Check sheet for the modelled part. Datum: model origin and axes. Units: mm. Coordinates: 2 decimals unless noted, no trailing zeros. Order: outer loops, then holes, each group sorted by start corner. A loop starts at its lowest first (then second) coordinate and runs counter-clockwise, first axis right, second up. Notation, with made-up numbers: (16.25, -34.5) -> (43.25, -34.5) arc R15 ccw to (43.25, -23.5) -> close; hole circle Ø1 at (26, 54.25). An arc over 180 degrees is marked (long way). Put each result on its own line as item: value. Start each with the question number.
Autodesk Inventor part; units mm, degrees
ref_plane "YZ Plane" through (0, 0, 0) normal (1, 0, 0) x (0, 1, 0)
ref_plane "XZ Plane" through (0, 0, 0) normal (0, 1, 0) x (-1, 0, 0)
ref_plane "XY Plane" through (0, 0, 0) normal (0, 0, 1) x (1, 0, 0)
sketch "Sketch1" plane through (0, 0, 0) normal (0, 0, 1) x (1, 0, 0)
  line L0 (0, -42.5799) -> (0, 42.5799)
  line L1 (-42.5799, 0) -> (42.5799, 0)
  line L2 (-28, 30) -> (28, 30)
  line L3 (30, 28) -> (30, -28)
  line L4 (28, -30) -> (-28, -30)
  line L5 (-30, -28) -> (-30, 28)
  arc A0 (-28, 30) -> (-30, 28) centre (-28, 28) ccw
  arc A1 (30, 28) -> (28, 30) centre (28, 28) ccw
  arc A2 (28, -30) -> (30, -28) centre (28, -28) ccw
  arc A3 (-30, -28) -> (-28, -30) centre (-28, -28) ccw
  circle A4 centre (0, 0) radius 23.5
  point P0 (-30, 30)
  point P1 (30, 30)
  point P2 (-22.4506, 22.4506)
  point P3 (-26.5, 15)
  point P4 (-15, 26.5)
  point P5 (-15, -26.5)
  point P6 (-22.4506, -22.4506)
  point P7 (-26.5, -15)
  point P8 (26.5, -15)
  point P9 (22.4506, -22.4506)
  point P10 (15, -26.5)
  point P11 (15, 26.5)
  point P12 (22.4506, 22.4506)
  point P13 (26.5, 15)
  point P14 (-21, 0)
  point P15 (21, 0)
  point P16 (-4.25, 0)
  point P17 (4.25, 0)
  point P18 (-24.6219, 5.3878)
  dimension "d0" = 60
  dimension "d1" = 2
  dimension "d2" = 22.4506
  dimension "d3" = 22.4506
  dimension "d4" = 15
  dimension "d5" = 15
  dimension "d6" = 3.5
  dimension "d7" = 3.5
  dimension "d10" = 360
  dimension "d28" = 9
  dimension "d36" = 25.75
  dimension "d48" = 47
extrude "Extrusion2" add sketch "Sketch1" along normal blind 3 contours L4 A3 L5 L1 A4 L0 | L0 A4 L1 L3 A2 L4 | L1 L5 A0 L2 L0 A4 | A4 L0 L2 A1 L3 L1
hole "Hole5" at (15, -26.5, 0) at (26.5, -15, 0) at (-15, -26.5, 0) at (-26.5, -15, 0) at (-26.5, 15, 0) at (-15, 26.5, 0) at (15, 26.5, 0) at (26.5, 15, 0) direction (0, 0, 1) diameter 2.4 end through all
hole "Hole6" at (-22.4506, 22.4506, 0) at (-22.4506, -22.4506, 0) at (22.4506, -22.4506, 0) at (22.4506, 22.4506, 0) direction (0, 0, 1) diameter 3.4 end through all
equation "\"d48\" = circle_dimension_inner"
equation "\"encoder_axis\" = 8"
equation "\"encoder_emboss\" = 0"
equation "\"encoders\" = 0"
equation "\"encoder_width\" = 27"
equation "\"front_plate_thickness\" = 2"
equation "\"glass_thickness\" = 2"
equation "\"screw_distance_outside\" = 3.5"
equation "\"encoder_rad\" = 49"
equation "\"encoder_extrude_hight\" = 3"
equation "\"screw_distance_center\" = 15"
equation "\"ring_top_thickness\" = 2"
equation "\"ring_outer_bevel_depth\" = 0.5"
equation "\"ring_depth\" = 6"
equation "\"ring_outer_bevel_height\" = 3"
equation "\"ring_inner_bevel_depth\" = 3.5"
equation "\"ring_thickness\" = 9"
equation "\"hole_from_center\" = 63.5"
equation "\"circle_dimension_inner\" = 47"
equation "\"circle_dimension\" = 56"
equation "\"backplate_width\" = 60"
equation "\"hole_distance\" = 22.45064"
properties part number "filler_ring-03" material "ABS Plastic"
1) Sectioned sample at C-C (x = -26.5). Record the boundary of the cut face in (y, z).
2) Sectioned sample at A-A (y = 0). Record the boundary of the cut face in (x, z), plus the area to 3 significant figures.
3) Scan lines: line 1 along X through (y, z) = (-26.5, 2); line 2 along Y through (x, z) = (0.5, 2). Record each from-to range of solid material in increasing order. Write a range as [from, to].
4) Mould release check, pull along Y, two halves, no side actions. Record for faces 1 (the cylindrical face through (16.17, 26.24, 1.52)), 2 (the flat face through (0, 30, 1)), 3 (the flat face through (-14, 20, 0)): +Y half, -Y half, draft (parallel to the pull), parting line (faces both ways), or undercut.
5) Sectioned sample at D-D (y = 15). Record the boundary of the cut face in (x, z), plus the area to 3 significant figures.
Entries:
1. outline: (-30, 0) -> (-16.2, 0) -> (-16.2, 3) -> (-30, 3) -> close; (-13.8, 0) -> (13.8, 0) -> (13.8, 3) -> (-13.8, 3) -> close; (16.2, 0) -> (30, 0) -> (30, 3) -> (16.2, 3) -> close
2. outline: (-30, 0) -> (-23.5, 0) -> (-23.5, 3) -> (-30, 3) -> close; (23.5, 0) -> (30, 0) -> (30, 3) -> (23.5, 3) -> close
2. area: 39.0 mm2
3. line 1: x = [-30, -16.2], [-13.8, 13.8], [16.2, 30]
3. line 2: y = [-30, -23.49], [23.49, 30]
4. face 1: undercut
4. face 2: +Y half
4. face 3: draft
5. outline: (-30, 0) -> (-27.7, 0) -> (-27.7, 3) -> (-30, 3) -> close; (-25.3, 0) -> (-18.09, 0) -> (-18.09, 3) -> (-25.3, 3) -> close; (18.09, 0) -> (25.3, 0) -> (25.3, 3) -> (18.09, 3) -> close; (27.7, 0) -> (30, 0) -> (30, 3) -> (27.7, 3) -> close
5. area: 57.1 mm2
